Check sheet for the modelled part. Datum: model origin and axes. Units: mm. A direction names the side the tool comes from. Coordinates: 2 decimals unless noted, no trailing zeros. Loops run counter-clockwise (first coordinate to the right, second up) from the corner with the lowest first, then second, coordinate; pieces in that order, holes last. Notation, with made-up numbers: (-5, 40.5) - (10, 40.5) arc R19 ccw to (10, 70.5) - close; hole circle Ø4 at (82.25, 88.25). An arc over 180 degrees is marked (long way). Write each question's results on one line, items separated by ' | '. Start each with the question number.
1. Cross-section at B-B (z = 0). Record the cut outline in (x, y), and give its area (3 significant figures).
2. Draft check along Y on faces 4 (the face through (10, 0, 0)), 5 (the face through (-7, -4, 2)), 6 (the face through (5, -2, 0)). Enter one of: released by +Y, released by -Y, zero draft, split by the parting line, or undercut.
3. Cross-section at C-C (x = 0). Record the cut outline in (y, z), and give its area (3 significant figures).
4. Cross-section at D-D (y = 1.25). Record the cut outline in (x, z), and give its area (3 significant figures).
5. Tool access check on faces 1 (the face through (-5, -3, -6.5)), 2 (the face through (3.5, -1.6, 0.1)), 3 (the face through (-5, -3, 6.5)). Record the directions out of +Z, -Z, +X, -X, +Y, -Y that give a thin tool (end or side, any length) a straight path to the whole face; none if there is none.
6. Thickness scan on line 1 (Y direction, x = 5.45, z = 0); line 2 (Z direction, x = 4.3, y = -3.5); line 3 (X direction, y = -4.5, z = -5). Record the ranges inside material, lowest first. Write a range as [from, to].
7. Cross-section at A-A (y = -3.5). Record the cut outline in (x, z), and give its area (3 significant figures).
8. Gauge pin test, flat ends, axial feed: P1, Ø3, axis at x = -1, y = 2.5, coming from the -Z side; P2, Ø6, axis at x = 15, z = -3, coming from the -Y side; P3, Ø4, axis at x = -4.5, y = -4, coming from the +Z side; P4, Ø4, axis at x = 10.5, y = -2.5, coming from the +Z side. Record the tip position at first contact, or that the pin passes through.
```python
from build123d import *

# Parameters (mm, degrees)
SKETCH1_R               = 22.5
BOSS_EXTRUDE1_DEPTH     = 4
SKETCH3_W               = 14
SKETCH3_H               = 11
BOSS_EXTRUDE2_DEPTH     = 6.5
SKETCH4_W               = 7
SKETCH4_H               = 14
CUT_EXTRUDE1_DEPTH      = 5
CUT_EXTRUDE1_DEPTH_BACK = 8
SKETCH5_R               = 1.5
CUT_EXTRUDE2_DEPTH      = 23.5
CUT_EXTRUDE2_DEPTH_BACK = 23.5


with BuildPart() as part:
    # Sketch1 → Boss-Extrude1 (new body)
    with BuildSketch(Plane(origin=(0, 0, 0), x_dir=(1, 0, 0), z_dir=(0, 1, 0))):
        Circle(SKETCH1_R)
    extrude(amount=BOSS_EXTRUDE1_DEPTH)

    # Sketch3 → Boss-Extrude2 (add, symmetric)
    with BuildSketch(Plane.XY):
        with Locations((0, -1.5)):
            Rectangle(SKETCH3_W, SKETCH3_H)
    extrude(amount=BOSS_EXTRUDE2_DEPTH, both=True)

    # Sketch4 → Cut-Extrude1 (cut, two sides)
    with BuildSketch(Plane(origin=(0, 0, 0), x_dir=(1, 0, 0), z_dir=(0, 1, 0))) as cut_extrude1_sk:
        Rectangle(SKETCH4_W, SKETCH4_H)
    extrude(amount=CUT_EXTRUDE1_DEPTH, mode=Mode.SUBTRACT)
    extrude(cut_extrude1_sk.sketch, amount=-CUT_EXTRUDE1_DEPTH_BACK, mode=Mode.SUBTRACT)

    # Sketch5 → Cut-Extrude2 (cut, two sides)
    with BuildSketch(Plane(origin=(0, 0, 0), x_dir=(0, 0, -1), z_dir=(1, 0, 0))) as cut_extrude2_sk:
        with Locations((0, -3.5)):
            Circle(SKETCH5_R)
    extrude(amount=CUT_EXTRUDE2_DEPTH, mode=Mode.SUBTRACT)
    extrude(cut_extrude2_sk.sketch, amount=-CUT_EXTRUDE2_DEPTH_BACK, mode=Mode.SUBTRACT)


solid = part.part
```
Established:
1) outline: (-22.5, 0) - (-7, 0) - (-7, -2) - (-3.5, -2) - (-3.5, 4) - (-22.5, 4) - close; (-7, -7) - (-3.5, -7) - (-3.5, -5) - (-7, -5) - close; (3.5, -7) - (7, -7) - (7, -5) - (3.5, -5) - close; (3.5, -2) - (7, -2) - (7, 0) - (22.5, 0) - (22.5, 4) - (3.5, 4) - close | area: 180 mm^2
2) face 4: released by -Y | face 5: zero draft | face 6: undercut
3) outline: (0, -22.5) - (4, -22.5) - (4, -7) - (0, -7) - close; (0, 7) - (4, 7) - (4, 22.5) - (0, 22.5) - close | area: 124 mm^2
4) outline: circle Ø45 at (0, 0); hole (-3.5, -7) - (3.5, -7) - (3.5, 7) - (-3.5, 7) - close | area: 1,490 mm^2
5) face 1: -Z, +X, -X, -Y | face 2: +Y, -Y | face 3: +Z, +X, -X, -Y
6) line 1: [-7, -5], [-2, 4] | line 2: [-6.5, -1.5], [1.5, 6.5] | line 3: [-7, -3.5], [3.5, 7]
7) outline: (-7, -6.5) - (-3.5, -6.5) - (-3.5, -1.5) - (-7, -1.5) - close; (-7, 1.5) - (-3.5, 1.5) - (-3.5, 6.5) - (-7, 6.5) - close; (3.5, -6.5) - (7, -6.5) - (7, -1.5) - (3.5, -1.5) - close; (3.5, 1.5) - (7, 1.5) - (7, 6.5) - (3.5, 6.5) - close | area: 70.0 mm^2
8) P1: z = -22.5 | P2: y = 0 | P3: z = 6.5 | P4: through
